Can you work these out from the model? Positions are in its coordinate system, mm. A direction names the side the tool comes from. Round coordinates to 2 decimals unless told otherwise and drop trailing zeros. Order: outer loops, then holes, each group sorted by start corner. A loop starts at its lowest first (then second) coordinate and runs counter-clockwise, first axis right, second up. Notation, with made-up numbers: (-29, 4) -> (-25, 4) arc R16 ccw to (-25, 19) -> close; hole circle Ø6 at (82.5, -10). An arc over 180 degrees is marked (long way). Use a Markdown table: item, result. Add a question column.
Q1. I'm going to push flat-ended pins straight in: pin 1 Ø0.7 at (x, z) = (9.5, -0.5) entering from -Y; pin 2 Ø1.2 at (x, z) = (3, 0.5) entering from -Y; pin 3 Ø4 at (x, y) = (-4, -4) entering from +Z. Where does each tip first touch, or does it pass through?
Q2. If we section it at C-C on x = -3: List the corners of the cut face in (y, z) for me, plus the area to 3 significant figures.
Q3. We'd pull the mould along X, two halves only. Please class faces 4 (the face through (-2.003, -3.448, -0.631)), 5 (the face through (-6, -3, 0)), 6 (the face through (2.619, -6.687, -2.432)): +X half, -X half, draft (parallel to the pull), parting line (faces both ways), or undercut.
Q4. If we section it at A-A on z = 0: List the corners of the cut face in (x, y) for me.
Q5. For faces 1 (the face through (2.4, -0.5, -4.3)), 2 (the face through (-4, -6.8, 0)), 3 (the face through (2.4, -0.5, 4.3)), which set-ups out of +Z, -Z, +X, -X, +Y, -Y let a thin tool reach every point of the face, with its end or its side?
Q6. I need wall thicknesses on line 1 along Z through (x, y) = (0, -3); line 2 along Y through (x, z) = (-4.5, -0.25); line 3 along Z through (x, y) = (2.5, -0.25). Which ranges of each line are inside material? Lowest first, please. Write a range as [from, to].
Q7. If we section it at B-B on y = -0.25: List the corners of the cut face in (x, z) for me.
Q8. If we section it at D-D on x = 0: List the corners of the cut face in (y, z) for me, plus the area to 3 significant figures.
```python
from build123d import *

# Parameters (mm, degrees)
BOSS_EXTRUDE1_DEPTH = 17
FILLET1_R           = 1
SKETCH2_W           = 2.35
SKETCH2_H           = 0.2
TAPPED_HOLE1_D      = 4.2


with BuildPart() as part:
    # Sketch1 → Boss-Extrude1 (new body)
    with BuildSketch(Plane(origin=(-6, 0, 0), x_dir=(0, 0, -1), z_dir=(1, 0, 0))):
        Polygon((3.9, 0), (-3.9, 0), (-3.9, -0.5), (-5.75, -0.5), (-5.75, -2), (-2.5, -6.8), (2.5, -6.8), (5.75, -2), (5.75, -0.5), (3.9, -0.5), align=None)
    extrude(amount=BOSS_EXTRUDE1_DEPTH)

    # Fillet1
    fillet1_edges = [part.edges().sort_by_distance(p)[0] for p in [
        (2.5, -0.5, 5.75),
        (2.5, -0.5, -5.75),
        (2.5, -2, -5.75),
        (2.5, -6.8, -2.5),
        (2.5, -6.8, 2.5),
        (2.5, -2, 5.75),
    ]]
    fillet(fillet1_edges, radius=FILLET1_R)

    # Sketch2 → Cut-Revolve1 (revolve, cut)
    with BuildSketch(Plane(origin=(7.5, 0, 0), x_dir=(0, 0, -1), z_dir=(1, 0, 0)), mode=Mode.PRIVATE) as cut_revolve1_sk:
        with Locations((1.175, -6.7)):
            Rectangle(SKETCH2_W, SKETCH2_H)
    revolve(cut_revolve1_sk.sketch.rotate(Axis((7.5, 1.665548573, 0), (0, -1, 0)), 180), axis=Axis((7.5, 1.665548573, 0), (0, -1, 0)), mode=Mode.SUBTRACT)

    # Sketch3 → Revolve1 (revolve)
    with BuildSketch(Plane(origin=(7.5, 0, 0), x_dir=(0, 0, -1), z_dir=(1, 0, 0)), mode=Mode.PRIVATE) as revolve1_sk:
        with BuildLine():
            Line((1.989974874, -6.6), (0, -6.6))
            Line((0, -6.6), (0, -7.8))
            ThreePointArc((0, -7.8), (1.161895004, -7.476784887), (1.989974874, -6.6))
        make_face()
    revolve(revolve1_sk.sketch.rotate(Axis((7.5, 0, 0), (0, -1, 0)), 180), axis=Axis((7.5, 0, 0), (0, -1, 0)))

    # Tapped Hole1 (through all)
    with Locations(Plane(origin=(0, 0, 0), x_dir=(1, 0, 0), z_dir=(0, 1, 0))):
        with Locations((0, 0)):
            Hole(TAPPED_HOLE1_D / 2)


solid = part.part
```
Answer below:
| question | item | result |
|---|---|---|
| 1 | pin 1 | y = -7.01 |
| 1 | pin 2 | y = -6.8 |
| 1 | pin 3 | z = 5.7 |
| 2 | outline | (-6.8, -1.97) arc R1 ccw to (-6.36, -2.8) -> (-2.25, -5.58) arc R1 ccw to (-1.69, -5.75) -> (-1.5, -5.75) arc R1 ccw to (-0.5, -4.75) -> (-0.5, -3.9) -> (0, -3.9) -> (0, 3.9) -> (-0.5, 3.9) -> (-0.5, 4.75) arc R1 ccw to (-1.5, 5.75) -> (-1.69, 5.75) arc R1 ccw to (-2.25, 5.58) -> (-6.36, 2.8) arc R1 ccw to (-6.8, 1.97) -> close |
| 2 | area | 60.2 mm² |
| 3 | face 4 | undercut |
| 3 | face 5 | -X half |
| 3 | face 6 | draft |
| 4 | outline | (-6, -6.8) -> (-2.1, -6.8) -> (-2.1, 0) -> (-6, 0) -> close; (2.1, -6.8) -> (5.15, -6.8) -> (5.15, -6.6) -> (5.51, -6.6) arc R2.25 ccw to (9.49, -6.6) -> (9.85, -6.6) -> (9.85, -6.8) -> (11, -6.8) -> (11, 0) -> (2.1, 0) -> close |
| 5 | face 1 | -Z, +X, -X, +Y |
| 5 | face 2 | +Z, -Z, -X, -Y |
| 5 | face 3 | +Z, +X, -X, +Y |
| 6 | line 1 | [-5.07, -2.1], [2.1, 5.07] |
| 6 | line 2 | [-6.8, 0] |
| 6 | line 3 | [-3.9, 3.9] |
| 7 | outline | (-6, -3.9) -> (11, -3.9) -> (11, 3.9) -> (-6, 3.9) -> close; hole circle Ø4.2 at (0, 0) |
| 8 | outline | (-6.79, -2.1) arc R1 ccw to (-6.36, -2.8) -> (-2.25, -5.58) arc R1 ccw to (-1.69, -5.75) -> (-1.5, -5.75) arc R1 ccw to (-0.5, -4.75) -> (-0.5, -3.9) -> (0, -3.9) -> (0, -2.1) -> close; (-6.79, 2.1) -> (0, 2.1) -> (0, 3.9) -> (-0.5, 3.9) -> (-0.5, 4.75) arc R1 ccw to (-1.5, 5.75) -> (-1.69, 5.75) arc R1 ccw to (-2.25, 5.58) -> (-6.36, 2.8) arc R1 ccw to start |
| 8 | area | 31.7 mm² |
